```python
from build123d import *

# Parameters (mm, degrees)
BOSS_EXTRUDE1_DEPTH = 7.62
SKETCH2_R           = 3.5
CUT_EXTRUDE1_DEPTH  = 8.62
SKETCH3_W           = 10.16
SKETCH3_H           = 7.62
BOSS_EXTRUDE2_DEPTH = 7.62


with BuildPart() as part:
    # Sketch1 → Boss-Extrude1 (new body)
    with BuildSketch(Plane(origin=(0, 0, 0), x_dir=(1, 0, 0), z_dir=(0, 1, 0))):
        with BuildLine():
            Line((0, 0), (0, 20))
            Line((0, 20), (32, 20))
            Line((32, 20), (32, 0))
            ThreePointArc((32, 0), (16, -16), (0, 0))
        make_face()
    extrude(amount=BOSS_EXTRUDE1_DEPTH)

    # Sketch2 → Cut-Extrude1 (cut, through all)
    with BuildSketch(Plane.XZ):
        with Locations((16, 0)):
            Circle(SKETCH2_R)
    extrude(amount=-CUT_EXTRUDE1_DEPTH, mode=Mode.SUBTRACT)

    # Sketch3 → Boss-Extrude2 (add)
    with BuildSketch(Plane(origin=(0, 0, -20), x_dir=(-1, 0, 0), z_dir=(0, 0, -1))):
        with Locations((-26.92, 3.81)):
            Rectangle(SKETCH3_W, SKETCH3_H)
        with Locations((-5.08, 3.81)):
            Rectangle(SKETCH3_W, SKETCH3_H)
    extrude(amount=BOSS_EXTRUDE2_DEPTH)


solid = part.part
```
Model file for the job. Use its own axes, mm. A direction names the side the tool comes from. Give positions to 0.01 mm unless a question says otherwise; leave off trailing zeros. Write each loop counter-clockwise with the first axis right and the second up, starting at its lowest first coordinate (ties: lowest second). Pieces come first, ordered by that corner, then holes. Notation, with made-up numbers: M 16.5,-8.75 L 39.5,-8.75 A18 cw 39.5,19.25 Z; hole C 18.25,-5 d10. An arc over 180 degrees is marked long. Use a Markdown table: item, result.
1) Pull direction X, two halves, no side cores. Call faces 1 (the cylindrical face through (16, 4, 16)), 2 (the flat face through (16, 4, -20)), 3 (the flat face through (10.16, 4, -24)), 4 (the flat face through (0, 4, -14)): +X half, -X half, draft (parallel to the pull), parting line (faces both ways), or undercut.
Responses:
| item | result |
|---|---|
| face 1 | parting line |
| face 2 | undercut |
| face 3 | undercut |
| face 4 | -X half |
2) Cut at B-B (y = 6.5). List the corners of the cut face in (x, z).
Responses:
| item | result |
|---|---|
| outline | M 0,-27.62 L 10.16,-27.62 L 10.16,-20 L 21.84,-20 L 21.84,-27.62 L 32,-27.62 L 32,0 A16 ccw 0,0 Z; hole C 16,0 d7 |
3) Pin check, flat tips, straight feed: pin 1 (6.5 mm diameter, centred on x = 16, z = 0, fed in from +Y); pin 2 (1 mm diameter, centred on y = 6, z = 1.5, fed in from +X); pin 3 (2 mm diameter, centred on x = 18.5, y = 5.5, fed in from -Z). Stop position of each tip, or through.
Responses:
| item | result |
|---|---|
| pin 1 | passes through |
| pin 2 | stops at x = 31.97 |
| pin 3 | stops at z = -20 |
4) Cut at A-A (x = 16). List the corners of the cut face in (y, z).
Responses:
| item | result |
|---|---|
| outline | M 0,-20 L 7.62,-20 L 7.62,-3.5 L 0,-3.5 Z; M 0,3.5 L 7.62,3.5 L 7.62,16 L 0,16 Z |
5) Cut at D-D (x = 22.5). List the corners of the cut face in (y, z), and give its area (3 significant figures).
Responses:
| item | result |
|---|---|
| outline | M 0,-27.62 L 7.62,-27.62 L 7.62,14.62 L 0,14.62 Z |
| area | 322 mm2 |
6) Cut at C-C (z = 4). List the corners of the cut face in (x, y), and give its area (3 significant figures).
Responses:
| item | result |
|---|---|
| outline | M 0.51,0 L 31.49,0 L 31.49,7.62 L 0.51,7.62 Z |
| area | 236 mm2 |
7) Drill centre lines: line 1 (Z direction, x = 16, y = 5.25); line 2 (Z direction, x = 14.5, y = 3.5); line 3 (Z direction, x = 8, y = 1.25). Where is each one in solid material? Low to high. Write a range as from..to.
Responses:
| item | result |
|---|---|
| line 1 | z = -20..-3.5, 3.5..16 |
| line 2 | z = -20..-3.16, 3.16..15.93 |
| line 3 | z = -27.62..13.86 |
8) Tool access for faces 5 (the flat face through (21.84, 4, -24)), 6 (the flat face through (16, 0, -6)): list every direction of +Z, -Z, +X, -X, +Y, -Y with a clear straight run to the whole face (end or side of a thin tool).
Responses:
| item | result |
|---|---|
| face 5 | -Z, +Y, -Y |
| face 6 | +Z, -Z, +X, -X, -Y |
